Part model, mm, in its own coordinate system. A direction names the side the tool comes from. Coordinates: 2 decimals unless noted, no trailing zeros. Write each loop counter-clockwise with the first axis right and the second up, starting at its lowest first coordinate (ties: lowest second). Pieces come first, ordered by that corner, then holes. Notation, with made-up numbers: (87, -19.75) - (146, -19.75) arc R30 cw to (146, 11.25) - close; hole circle Ø4 at (43, 80). An arc over 180 degrees is marked (long way). Use a Markdown table: item, result.
```python
from build123d import *

# Parameters (mm, degrees)
EXTRUDE_3_DEPTH          = 120
SKETCH_4_R               = 4
SKETCH_4_W               = 14
SKETCH_4_H               = 11
CUT_EXTRUDE_1_DEPTH      = 120
CUT_EXTRUDE_2_DEPTH      = 5
SKETCH_5_W               = 23
SKETCH_5_H               = 7
CUT_EXTRUDE_3_DEPTH      = 98
SKETCH_6_W               = 100
SKETCH_6_H               = 53.539105243
CUT_EXTRUDE_4_DEPTH      = 98
SKETCH_7_R               = 1.4
CUT_EXTRUDE_5_DEPTH      = 5
SKETCH_13_W              = 16
SKETCH_13_H              = 16
SKETCH_13_R              = 3
EXTRUDE_8_DEPTH          = 10
CUT_EXTRUDE_7_DEPTH      = 155.609184721
CUT_EXTRUDE_7_DEPTH_BACK = 155.609184721
SKETCH_15_R              = 2.1


with BuildPart() as part:
    # Эскиз3 → Бобышка-Вытянуть3 (new body)
    with BuildSketch(Plane(origin=(0, 0, 0), x_dir=(0, 0, -1), z_dir=(1, 0, 0))):
        Polygon((0, 0), (52, 0), (52, 52), align=None)
    extrude(amount=EXTRUDE_3_DEPTH)

    # Эскиз4 → Вырез-Вытянуть1 (cut)
    with BuildSketch(Plane(origin=(0, 0, 0), x_dir=(1, 0, 0), z_dir=(0, 0.7071067811865477, 0.7071067811865475))):
        with Locations(Location((70, 36.5, 0), (0, 0, 270))):
            Circle(SKETCH_4_R)
        with Locations((95, 36.5)):
            Rectangle(SKETCH_4_W, SKETCH_4_H)
    extrude(amount=-CUT_EXTRUDE_1_DEPTH, mode=Mode.SUBTRACT)

    # Эскиз4<3> → Вырез-Вытянуть2 (cut)
    with BuildSketch(Plane(origin=(0, 0, 0), x_dir=(1, 0, 0), z_dir=(0, 0.7071067811865477, 0.7071067811865475))):
        Polygon((48, 58), (48, 65), (25, 65), (25, 58), (15, 58), (15, 15), (55, 15), (55, 58), align=None)
    extrude(amount=-CUT_EXTRUDE_2_DEPTH, mode=Mode.SUBTRACT)

    # Эскиз5 → Вырез-Вытянуть3 (cut)
    with BuildSketch(Plane(origin=(0, -3.535533906, -3.535533906), x_dir=(1, 0, 0), z_dir=(0, 0.7071067811865477, 0.7071067811865474))):
        with Locations((36.5, 61.5)):
            Rectangle(SKETCH_5_W, SKETCH_5_H)
    extrude(amount=-CUT_EXTRUDE_3_DEPTH, mode=Mode.SUBTRACT)

    # Эскиз6 → Вырез-Вытянуть4 (cut)
    with BuildSketch(Plane(origin=(0, -7.071067812, -7.071067812), x_dir=(1, 0, 0), z_dir=(0, 0.7071067811865477, 0.7071067811865474))):
        with Locations((60, 36.769552621)):
            Rectangle(SKETCH_6_W, SKETCH_6_H)
    extrude(amount=-CUT_EXTRUDE_4_DEPTH, mode=Mode.SUBTRACT)

    # Эскиз7 → Вырез-Вытянуть5 (cut)
    with BuildSketch(Plane(origin=(0, 0, 0), x_dir=(1, 0, 0), z_dir=(0, 0.7071067811865477, 0.7071067811865475))):
        with Locations(Location((10, 63.539105243, 0), (0, 0, 270))):
            Circle(SKETCH_7_R)
        with Locations(Location((110, 10, 0), (0, 0, 270))):
            Circle(SKETCH_7_R)
        with Locations(Location((110, 63.539105243, 0), (0, 0, 270))):
            Circle(SKETCH_7_R)
        with Locations(Location((10, 10, 0), (0, 0, 270))):
            Circle(SKETCH_7_R)
    extrude(amount=-CUT_EXTRUDE_5_DEPTH, mode=Mode.SUBTRACT)

    # Эскиз13 → Бобышка-Вытянуть8 (add)
    # profile 1 of 2: a face of its own
    with BuildSketch(Plane(origin=(0, 0, 0), x_dir=(-1, 0, 0), z_dir=(0, -1, 0))):
        with Locations((-128, 44)):
            Rectangle(SKETCH_13_W, SKETCH_13_H)
        with Locations(Location((-128, 44, 0), (0, 0, 90))):
            Circle(SKETCH_13_R, mode=Mode.SUBTRACT)
    # profile 2 of 2: a face of its own
    with BuildSketch(Plane(origin=(0, 0, 0), x_dir=(-1, 0, 0), z_dir=(0, -1, 0))):
        with Locations((8, 44)):
            Rectangle(SKETCH_13_W, SKETCH_13_H)
        with Locations(Location((8, 44, 0), (0, 0, 90))):
            Circle(SKETCH_13_R, mode=Mode.SUBTRACT)
    extrude(amount=-EXTRUDE_8_DEPTH)

    # Эскиз15 → Вырез-Вытянуть7 (cut, two sides: drawn at the far end of the back side and taken through both)
    with BuildSketch(Plane.ZY.offset(-CUT_EXTRUDE_7_DEPTH_BACK)):
        with Locations(Location((-27.888881523, 8.434002899, 0), (0, 0, 90))):
            Circle(SKETCH_15_R)
    extrude(amount=CUT_EXTRUDE_7_DEPTH + CUT_EXTRUDE_7_DEPTH_BACK, mode=Mode.SUBTRACT)


solid = part.part
```
Item 1: Two-plate mould, pull along X, no slides. Class faces 4 (the face through (-16, 5, -44)), 5 (the face through (20.07, 39.269, -42.755)), 6 (the face through (59, 26, -26)): pulls with the +X half, pulls with the -X half, needs draft (parallel to the pull), parting line crosses it, or undercut.
From the geometry:
| item | result |
|---|---|
| face 4 | pulls with the -X half |
| face 5 | undercut |
| face 6 | needs draft |
Item 2: Which spindle directions (+Z, -Z, +X, -X, +Y, -Y) get a long thin tool onto all of the face, cutting with end or side? Do faces 1 (the face through (51.549, 39.269, -42.755)), 2 (the face through (36.339, 35.734, -46.291)), 3 (the face through (102, 22, -29)). Say none if no direction does.
From the geometry:
| item | result |
|---|---|
| face 1 | +Z |
| face 2 | -Z |
| face 3 | none |
Item 3: Band-saw the part on D-D, the plane z = -16. Give the cut face in (x, y), then the cut area to 3 significant figures.
From the geometry:
| item | result |
|---|---|
| outline | (0, 0) - (10, 0) - (10, 1.86) - (110, 1.86) - (110, 0) - (120, 0) - (120, 16) - (55, 16) - (55, 8.93) - (15, 8.93) - (15, 16) - (0, 16) - close |
| area | 1,450 mm^2 |
Item 4: Drill centre lines: probe 1 along X at (y, z) = (4.5, -44); probe 2 along X at (y, z) = (12, -29); probe 3 along Z at (x, y) = (128, 6). Where is each one in solid material? Low to high.
From the geometry:
| item | result |
|---|---|
| probe 1 | -16 to -11, -5 to 10, 110 to 125, 131 to 136 |
| probe 2 | 0 to 10, 110 to 120 |
| probe 3 | -52 to -47, -41 to -36 |
Item 5: Band-saw the part on A-A, the plane x = -8. Give the cut face in (y, z), then the cut area to 3 significant figures.
From the geometry:
| item | result |
|---|---|
| outline | (0, -52) - (10, -52) - (10, -47) - (0, -47) - close; (0, -41) - (10, -41) - (10, -36) - (0, -36) - close |
| area | 100 mm^2 |
Item 6: Band-saw the part on B-B, the plane x = 20.5. Give the cut face in (y, z).
From the geometry:
| item | result |
|---|---|
| outline | (0, -14.14) - (37.86, -52) - (52, -52) - (41.01, -41.01) - (37.48, -44.55) - (7.07, -14.14) - (10.61, -10.61) - (0, 0) - close |
Item 7: Band-saw the part on C-C, the plane x = 40.5. Give the cut face in (y, z).
From the geometry:
| item | result |
|---|---|
| outline | (0, -14.14) - (33.94, -48.08) - (37.48, -44.55) - (7.07, -14.14) - (10.61, -10.61) - (0, 0) - close; (39.92, -52) - (52, -52) - (45.96, -45.96) - close |
Item 8: Drop flat-ended pins along their axis: P1, Ø1.5, axis at y = 31.5, z = -37.5, coming from the +X side; P2, Ø8, axis at x = 59, y = 32, coming from the -Z side; P3, Ø3.5, axis at x = -8, z = -44, coming from the +Y side; P4, Ø7.5, axis at y = 23.5, z = -28.5, coming from the -X side. Give the stop position or say it passes through.
From the geometry:
| item | result |
|---|---|
| P1 | x = 120 |
| P2 | z = -50.14 |
| P3 | through |
| P4 | x = 0 |
